The model under review builds one solid part; all positions refer to its coordinate system, in mm. A direction names the side the tool comes from. Give positions to 0.01 mm unless a question says otherwise; leave off trailing zeros. Order: outer loops, then holes, each group sorted by start corner. A loop starts at its lowest first (then second) coordinate and runs counter-clockwise, first axis right, second up.
Autodesk Inventor part; units mm, degrees
ref_plane "YZ Plane" through (0, 0, 0) normal (1, 0, 0) x (0, 1, 0)
ref_plane "XZ Plane" through (0, 0, 0) normal (0, 1, 0) x (-1, 0, 0)
ref_plane "XY Plane" through (0, 0, 0) normal (0, 0, 1) x (1, 0, 0)
sketch "スケッチ1" plane through (0, 0, 0) normal (0, 1, 0) x (-1, 0, 0)
  point P0 (0, 0)
sketch "スケッチ2" plane through (0, 0, 0) normal (0, 0, 1) x (1, 0, 0)
  circle A0 centre (0, 0) radius 3.5
  circle A1 centre (0, 0) radius 7.5
  line L0 (0, 0) -> (0, -152.95)
  circle A2 centre (0, -152.95) radius 3.5
  circle A3 centre (0, -152.95) radius 7.5
  line L1 (7.5, -152.95) -> (7.5, 0)
  line L2 (-7.5, 0) -> (-7.5, -152.95)
  dimension "d0" = 7
  dimension "d1" = 15
  dimension "d2" = 152.95
  dimension "d3" = 7
  dimension "d4" = 15
extrude "押し出し1" add sketch "スケッチ2" along normal blind 4
sketch "スケッチ4" plane through (0, 0, 4) normal (0, 0, 1) x (1, 0, 0)
  arc A0 (7.5, 0) -> (-7.5, 0) centre (0, 0) ccw
  circle A1 centre (0, 0) radius 4.25
  circle A2 centre (0, -152.95) radius 3.5
  circle A3 centre (0, -152.95) radius 4.25
  dimension "d10" = 8.5
  dimension "d11" = 8.5
extrude "押し出し3" cut sketch "スケッチ4" against normal blind 2
properties part number "motor_holder_top"
Item 1: Clearance check with flat-ended pins moving along their axes: pin 1 Ø4 at (x, y) = (1.5, -1) entering from +Z; pin 2 Ø1 at (x, z) = (3.5, 3) entering from +Y. State where each tip first meets the part, or that it passes through.
Values found:
pin 1: stops at z = 2
pin 2: stops at y = 6.87
Item 2: Draft analysis for pull direction X (two halves, no side actions). For faces 1 (the cylindrical face through (-0.92, -157.1, 3.01)), 2 (the flat face through (-7.5, -75, 2)), 3 (the cylindrical face through (-0.16, 7.5, 1.97)), state which applies: released by +X, released by -X, zero draft, split by the parting line, or undercut.
Values found:
face 1: undercut
face 2: released by -X
face 3: split by the parting line
Item 3: Take a section at B-B (z = 3.25). Give the boundary of the cut face in (x, y).
Values found:
outline: (-7.5, -152.95) arc R7.5 ccw to (7.5, -152.95) - (7.5, 0) arc R7.5 ccw to (-7.5, 0) - close; hole circle Ø8.5 at (0, -152.95); hole circle Ø8.5 at (0, 0)
Item 4: For faces 4 (the cylindrical face through (0.16, -160.45, 1.97)), 5 (the flat face through (1, -149, 2)), list the 3-axis set-ups (+Z, -Z, +X, -X, +Y, -Y) from which the entire face can be reached by the end or side of a thin tool; tool diameter is ignored.
Values found:
face 4: +Z, -Z, -Y
face 5: +Z
Item 5: For line 1 (Y direction, x = 0, z = 1.2); line 2 (Y direction, x = 0, z = 2.6); line 3 (X direction, y = 0, z = 0.65), list the stretches that pass through material, from the lowest coordinate up.
Values found:
line 1: y = -160.45 to -156.45, -149.45 to -3.5, 3.5 to 7.5
line 2: y = -160.45 to -157.2, -148.7 to -4.25, 4.25 to 7.5
line 3: x = -7.5 to -3.5, 3.5 to 7.5
Item 6: Take a section at A-A (x = 0). Give the boundary of the cut face in (y, z).
Values found:
outline: (-160.45, 0) - (-156.45, 0) - (-156.45, 2) - (-157.2, 2) - (-157.2, 4) - (-160.45, 4) - close; (-149.45, 0) - (-3.5, 0) - (-3.5, 2) - (-4.25, 2) - (-4.25, 4) - (-148.7, 4) - (-148.7, 2) - (-149.45, 2) - close; (3.5, 0) - (7.5, 0) - (7.5, 4) - (4.25, 4) - (4.25, 2) - (3.5, 2) - close
